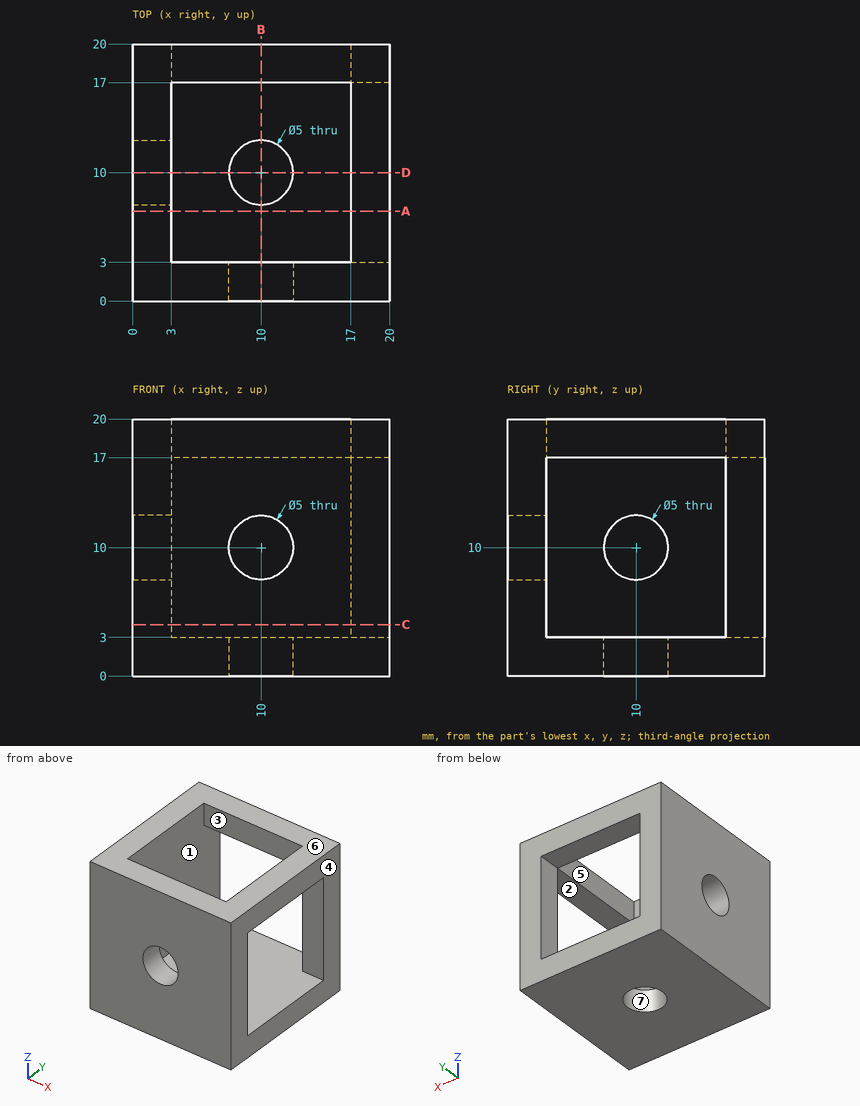
The drawing under review shows one solid part. Ordinate dimensions are in mm from its lowest x, y, z. A direction names the side the tool comes from. Coordinates: 2 decimals unless noted, no trailing zeros. Order: outer loops, then holes, each group sorted by start corner. A loop starts at its lowest first (then second) coordinate and runs counter-clockwise, first axis right, second up. Notation, with made-up numbers: (-14.75, -17.5) - (41.25, -17.5) arc R31 cw to (41.25, 20.5) - close; hole circle Ø8 at (23.5, -35.5). An arc over 180 degrees is marked (long way). Put each result on its own line as item: value.
1) Tool access review of the marked faces 1, 2 and 3: name each direction out of +Z, -Z, +X, -X, +Y, -Y from which nothing blocks a thin tool from reaching the whole face with its end or side.
Response values:
face 1: none
face 2: +X
face 3: +Z
2) Take a section at B-B, the plane x = 10. Give the boundary of the cut face in (y, z).
Response values:
outline: (0, 0) - (7.5, 0) - (7.5, 3) - (3, 3) - (3, 7.5) - (0, 7.5) - close; (0, 12.5) - (3, 12.5) - (3, 20) - (0, 20) - close; (12.5, 0) - (20, 0) - (20, 3) - (12.5, 3) - close; (17, 17) - (20, 17) - (20, 20) - (17, 20) - close
3) Take a section at A-A, the plane y = 7. Give the boundary of the cut face in (x, z), and give its area (3 significant figures).
Response values:
outline: (0, 0) - (20, 0) - (20, 3) - (3, 3) - (3, 20) - (0, 20) - close; (17, 17) - (20, 17) - (20, 20) - (17, 20) - close
area: 120 mm²
4) Insertion check: P1, Ø3, axis at x = 7.5, z = 8, coming from the +Y side; P2, Ø5, axis at y = 13.5, z = 9.5, coming from the +X side; P3, Ø3, axis at x = 14.5, y = 14, coming from the +Z side. Each pin has a flat end and moves straight along its axis. Give the tip position at first contact, or say it passes through.
Response values:
P1: stops at y = 3
P2: stops at x = 3
P3: stops at z = 3
5) Wall thickness on L1, parallel to Z at x = 1.2, y = 10; L2, parallel to X at y = 17.75, z = 12: over which ranges is each line inside the solid? List them lowest first. Write a range as from..to.
Response values:
L1: z = 0..7.5, 12.5..20
L2: x = 0..3, 17..20
6) The part is to be moulded in two halves that separate along X. For the marked faces 4, 5, 6 and 7, say which applies: released by +X, released by -X, zero draft, split by the parting line, or undercut.
Response values:
face 4: released by +X
face 5: undercut
face 6: zero draft
face 7: undercut
